Can you work these out from the drawing? Everything is in mm from the part's minimum corner. A direction names the side the tool comes from. Coordinates: 2 decimals unless noted, no trailing zeros. Order: outer loops, then holes, each group sorted by start corner. A loop starts at its lowest first (then second) coordinate and runs counter-clockwise, first axis right, second up. Notation, with made-up numbers: (9.5, 12.5) -> (59.5, 12.5) arc R21 cw to (59.5, 26.5) -> close; hole circle Ø10 at (-21.75, 44). An arc over 180 degrees is marked (long way). Put each result on its own line as item: value. Start each with the question number.
Q1. If we section it at A-A (x = 28): Please give me the cut outline in (y, z).
Q2. We'd pull the mould along Y, two halves only. Please class the marked faces 1, 2 and 3: +Y half, -Y half, draft (parallel to the pull), parting line (faces both ways), or undercut.
Q3. Will these pins go through, and if not, where does the flat tip stop? pin 1 (19 mm diameter, centred on x = 28, y = 28, fed in from -Z); pin 2 (10.5 mm diameter, centred on x = 28, y = 28, fed in from -Z); pin 3 (1 mm diameter, centred on x = 22, z = 24, fed in from -Y); pin 4 (6 mm diameter, centred on x = 27.5, z = 11, fed in from -Y).
Q4. Please list where these lines run through material, in increasing order: line 1 along Z through (x, y) = (11, 33.5); line 2 along Y through (x, z) = (28, 17.25); line 3 along X through (y, z) = (21.5, 25).
Q5. If we section it at D-D (y = 37): Please give me the cut outline in (x, z), and give its area (3 significant figures).
Q6. If we section it at C-C (z = 23.75): Please give me the cut outline in (x, y).
Q7. For the marked faces 4, 5 and 6, which set-ups out of +Z, -Z, +X, -X, +Y, -Y let a thin tool reach every point of the face, with its end or its side?
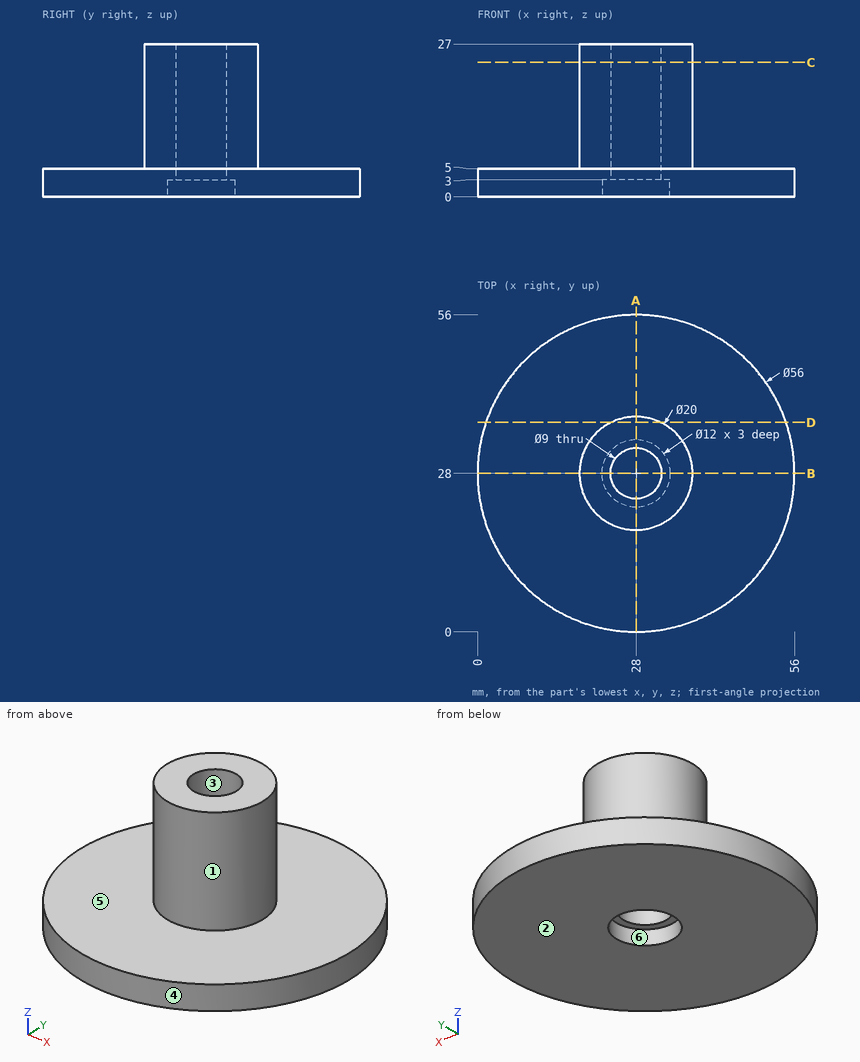
The answers:
1. outline: (0, 0) -> (22, 0) -> (22, 3) -> (23.5, 3) -> (23.5, 27) -> (18, 27) -> (18, 5) -> (0, 5) -> close; (32.5, 3) -> (34, 3) -> (34, 0) -> (56, 0) -> (56, 5) -> (38, 5) -> (38, 27) -> (32.5, 27) -> close
2. face 1: parting line
2. face 2: draft
2. face 3: undercut
3. pin 1: z = 0
3. pin 2: z = 3
3. pin 3: y = 19.65
3. pin 4: y = 18
4. line 1: 0 to 5
4. line 2: 18 to 23.5, 32.5 to 38
4. line 3: 20.4 to 35.6
5. outline: (1.49, 0) -> (54.51, 0) -> (54.51, 5) -> (32.36, 5) -> (32.36, 27) -> (23.64, 27) -> (23.64, 5) -> (1.49, 5) -> close
5. area: 457 mm^2
6. outline: circle Ø20 at (28, 28); hole circle Ø9 at (28, 28)
7. face 4: +Z, -Z
7. face 5: +Z
7. face 6: -Z
